Could you check a few things on this drawing? It's one solid part, dimensions in mm from its lowest x, y, z. A direction names the side the tool comes from. Coordinates: 2 decimals unless noted, no trailing zeros. Write each loop counter-clockwise with the first axis right and the second up, starting at its lowest first coordinate (ties: lowest second). Pieces come first, ordered by that corner, then holes. Notation, with made-up numbers: M 89.25,-29.75 L 105.25,-29.75 A24 ccw 105.25,-13.75 Z; hole C 88,53.5 d3. An arc over 180 degrees is marked long. Use a Markdown table: item, result.
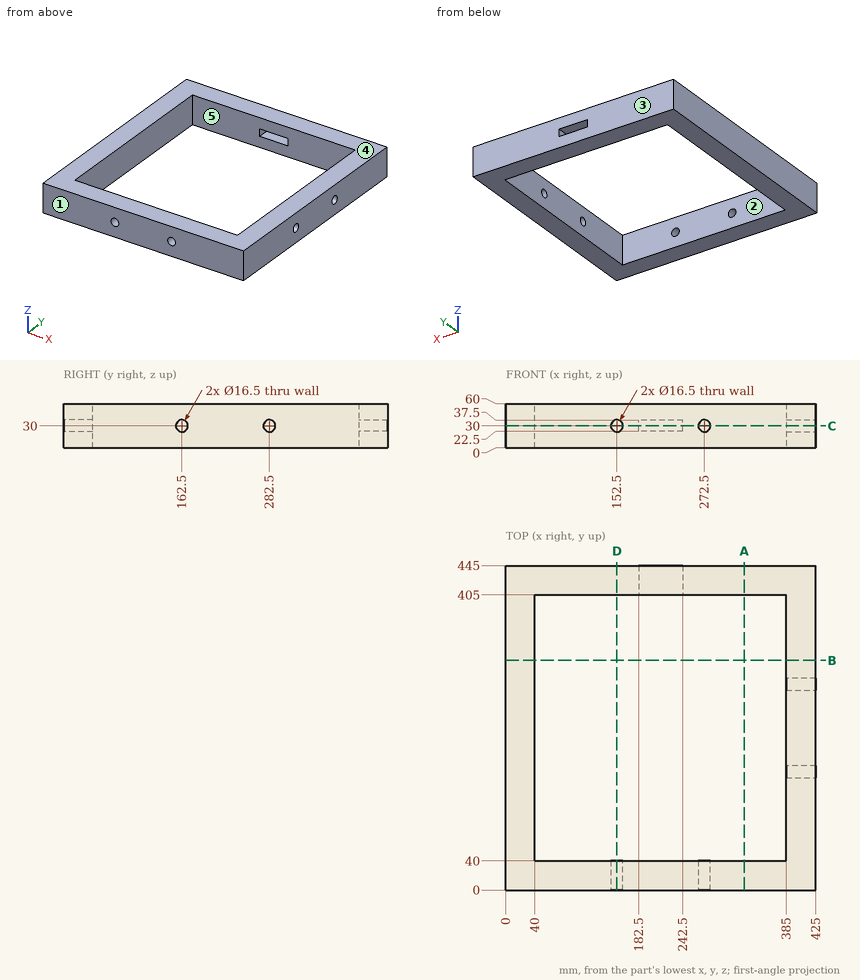
1. Suppose I cut it at A-A on x = 327.5. Write out the boundary of the cut face in (y, z), and give its area (3 significant figures).
Answers follow:
| item | result |
|---|---|
| outline | M 0,0 L 40,0 L 40,60 L 0,60 Z; M 405,0 L 445,0 L 445,60 L 405,60 Z |
| area | 4,800 mm2 |
2. Which directions (+Z, -Z, +X, -X, +Y, -Y) give clear straight access to the entire face, cutting with the end or side of a thin tool? Please do the marked faces 4 and 5.
Answers follow:
| item | result |
|---|---|
| face 4 | +Z, +X, -X, +Y, -Y |
| face 5 | +Z, -Z |
3. I need wall thicknesses on probe 1 along Y at (x, z) = (284, 47); probe 2 along Y at (x, z) = (386.5, 32); probe 3 along X at (y, z) = (335, 40). Which ranges of each line are inside material? Lowest first, please.
Answers follow:
| item | result |
|---|---|
| probe 1 | y = 0 to 40, 405 to 445 |
| probe 2 | y = 0 to 154.5, 170.5 to 274.5, 290.5 to 445 |
| probe 3 | x = 0 to 40, 385 to 425 |
4. Suppose I cut it at B-B on y = 315. Write out the boundary of the cut face in (x, z), and give its area (3 significant figures).
Answers follow:
| item | result |
|---|---|
| outline | M 0,0 L 40,0 L 40,60 L 0,60 Z; M 385,0 L 425,0 L 425,60 L 385,60 Z |
| area | 4,800 mm2 |
5. Suppose I cut it at C-C on z = 30. Write out the boundary of the cut face in (x, y).
Answers follow:
| item | result |
|---|---|
| outline | M 0,0 L 144.25,0 L 144.25,40 L 40,40 L 40,405 L 182.5,405 L 182.5,445 L 0,445 Z; M 160.75,0 L 264.25,0 L 264.25,40 L 160.75,40 Z; M 242.5,405 L 385,405 L 385,290.75 L 425,290.75 L 425,445 L 242.5,445 Z; M 280.75,0 L 425,0 L 425,154.25 L 385,154.25 L 385,40 L 280.75,40 Z; M 385,170.75 L 425,170.75 L 425,274.25 L 385,274.25 Z |
6. We'd pull the mould along Y, two halves only. Please class the marked faces 1, 2 and 3: +Y half, -Y half, draft (parallel to the pull), parting line (faces both ways), or undercut.
Answers follow:
| item | result |
|---|---|
| face 1 | -Y half |
| face 2 | undercut |
| face 3 | +Y half |
7. Suppose I cut it at D-D on x = 152.5. Write out the boundary of the cut face in (y, z).
Answers follow:
| item | result |
|---|---|
| outline | M 0,0 L 40,0 L 40,21.75 L 0,21.75 Z; M 0,38.25 L 40,38.25 L 40,60 L 0,60 Z; M 405,0 L 445,0 L 445,60 L 405,60 Z |
